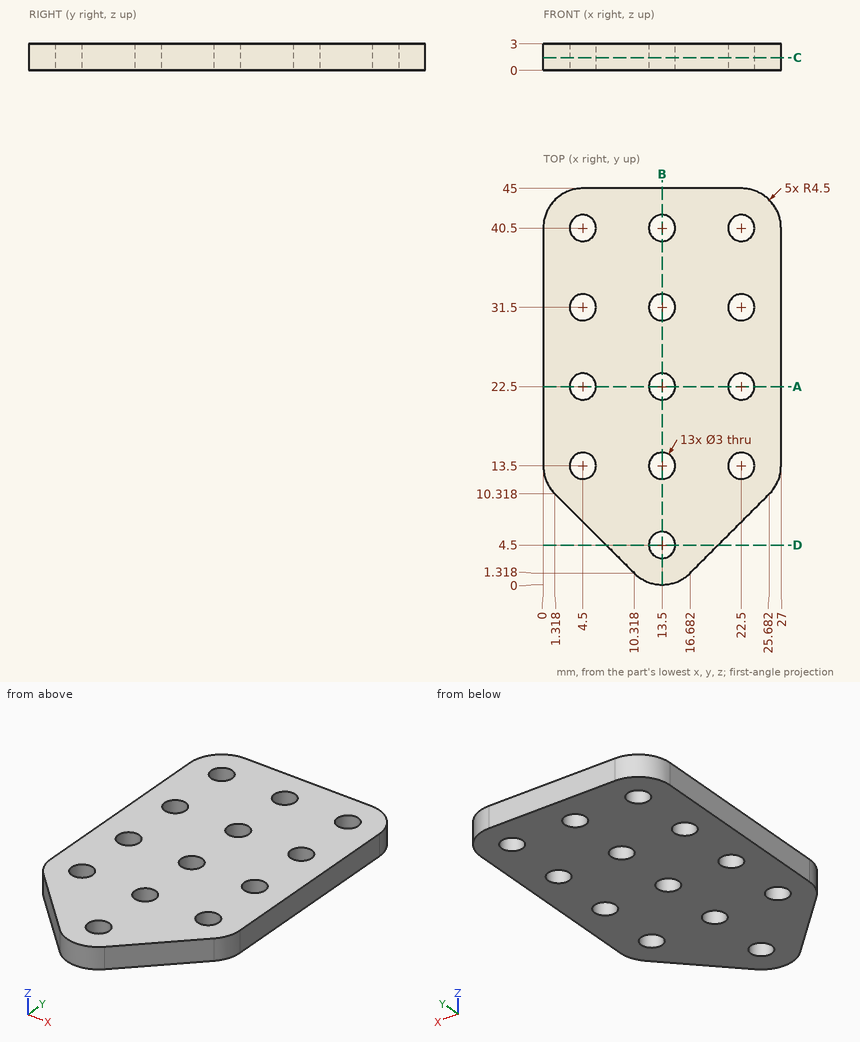
Drawing for the job (mm, zero at the part's lowest x, y, z). Round coordinates to 2 decimals unless told otherwise and drop trailing zeros. Order: outer loops, then holes, each group sorted by start corner. A loop starts at its lowest first (then second) coordinate and runs counter-clockwise, first axis right, second up. Notation, with made-up numbers: M 72,21 L 76,21 A21 ccw 76,46 Z; hole C 86.5,-37.5 d10. An arc over 180 degrees is marked long. Use one line per item in the form item = value.
Q1. Probe L1, parallel to Y at x = 13.5, z = 0.9; L2, parallel to X at y = 31.5, z = 1.6; L3, parallel to Y at x = 4, z = 0.2. List the from-to ranges inside material, lowest first.
Recorded:
L1 = 0 to 3, 6 to 12, 15 to 21, 24 to 30, 33 to 39, 42 to 45
L2 = 0 to 3, 6 to 12, 15 to 21, 24 to 27
L3 = 7.64 to 12.09, 14.91 to 21.09, 23.91 to 30.09, 32.91 to 39.09, 41.91 to 44.97
Q2. Saw through at C-C on z = 1.45. State how many separate pieces and enclosed holes the cut face has, then the cut area to 3 significant figures.
Recorded:
separate_pieces = 1
enclosed_holes = 13
area = 977 mm^2
Q3. Saw through at D-D on y = 4.5. Give the cut face in (x, z).
Recorded:
outline = M 7.14,0 L 12,0 L 12,3 L 7.14,3 Z; M 15,0 L 19.86,0 L 19.86,3 L 15,3 Z
Q4. Saw through at A-A on y = 22.5. Give the cut face in (x, z), then the cut area to 3 significant figures.
Recorded:
outline = M 0,0 L 3,0 L 3,3 L 0,3 Z; M 6,0 L 12,0 L 12,3 L 6,3 Z; M 15,0 L 21,0 L 21,3 L 15,3 Z; M 24,0 L 27,0 L 27,3 L 24,3 Z
area = 54.0 mm^2
Q5. Saw through at B-B on x = 13.5. Give the cut face in (y, z).
Recorded:
outline = M 0,0 L 3,0 L 3,3 L 0,3 Z; M 6,0 L 12,0 L 12,3 L 6,3 Z; M 15,0 L 21,0 L 21,3 L 15,3 Z; M 24,0 L 30,0 L 30,3 L 24,3 Z; M 33,0 L 39,0 L 39,3 L 33,3 Z; M 42,0 L 45,0 L 45,3 L 42,3 Z
Q6. Flat gauge pin, fed straight in: P1, Ø1.5, axis at x = 24, z = 2.5, coming from the +Y side. Where does the tip first touch, or does it go through?
Recorded:
P1 = 44.94
